Work out the finished part from the listing and answer in its coordinate system (mm). Face numbers are marked on the shaded views. A direction names the side the tool comes from. Give positions to 0.01 mm unless a question says otherwise; leave off trailing zeros. Loops run counter-clockwise (first coordinate to the right, second up) from the corner with the lowest first, then second, coordinate; pieces in that order, holes last. Notation, with made-up numbers: M 4,20.25 L 49,20.25 A24 cw 49,47.25 Z; hole C -7,43.25 d10. An arc over 180 degrees is marked long. Use a Markdown table: item, result.
```python
from build123d import *

# Parameters (mm, degrees)
CROQUIS1_W              = 70
CROQUIS1_H              = 42
SALIENTE_EXTRUIR1_DEPTH = 28
CROQUIS2_W              = 1.5
CROQUIS2_H              = 19.5
CORTAR_EXTRUIR1_DEPTH   = 70
CROQUIS3_R              = 2
CORTAR_EXTRUIR2_DEPTH   = 70
CROQUIS4_R              = 6
CORTAR_EXTRUIR3_DEPTH   = 70
CROQUIS5_R              = 10.4
CORTAR_EXTRUIR4_DEPTH   = 4.5
CROQUIS6_R              = 9.7
CROQUIS6_R_2            = 6.7
CORTAR_EXTRUIR5_DEPTH   = 1
CHAFL_N1_SIZE           = 1.2
REDONDEO1_R             = 0.7


with BuildPart() as part:
    # Croquis1 → Saliente-Extruir1 (new body)
    with BuildSketch(Plane.XY):
        Rectangle(CROQUIS1_W, CROQUIS1_H)
    extrude(amount=SALIENTE_EXTRUIR1_DEPTH)

    # Croquis2 → Cortar-Extruir1 (cut)
    with BuildSketch(Plane(origin=(35, 0, 0), x_dir=(0, 0, -1), z_dir=(1, 0, 0))):
        with Locations((-27.25, 0)):
            Rectangle(CROQUIS2_W, CROQUIS2_H)
        Polygon((0, 21), (-20, 21), (-20, 19.5), (-4.5, 19.5), (-4.5, 10.5), (0, 6), align=None)
        Polygon((-20, -19.5), (-20, -21), (0, -21), (0, -6), (-4.5, -10.5), (-4.5, -19.5), align=None)
    extrude(amount=-CORTAR_EXTRUIR1_DEPTH, mode=Mode.SUBTRACT)

    # Croquis3 → Cortar-Extruir2 (cut)
    with BuildSketch(Plane.XY.offset(28)):
        with Locations((25, -15)):
            Circle(CROQUIS3_R)
        with Locations((-25, -15)):
            Circle(CROQUIS3_R)
        with Locations((-25, 15)):
            Circle(CROQUIS3_R)
        with Locations((25, 15)):
            Circle(CROQUIS3_R)
    extrude(amount=-CORTAR_EXTRUIR2_DEPTH, mode=Mode.SUBTRACT)

    # Croquis4 → Cortar-Extruir3 (cut)
    with BuildSketch(Plane(origin=(35, 0, 0), x_dir=(0, 0, -1), z_dir=(1, 0, 0))):
        with Locations((-13, 0)):
            Circle(CROQUIS4_R)
    extrude(amount=-CORTAR_EXTRUIR3_DEPTH, mode=Mode.SUBTRACT)

    # Croquis5 → Cortar-Extruir4 (cut)
    with BuildSketch(Plane(origin=(35, 0, 0), x_dir=(0, 0, -1), z_dir=(1, 0, 0))):
        with Locations((-13, 0)):
            Circle(CROQUIS5_R)
    cortar_extruir4 = extrude(amount=-CORTAR_EXTRUIR4_DEPTH, mode=Mode.SUBTRACT)

    # Croquis6 → Cortar-Extruir5 (cut)
    with BuildSketch(Plane(origin=(30.5, 0, 0), x_dir=(0, 0, -1), z_dir=(1, 0, 0))):
        with Locations((-13, 0)):
            Circle(CROQUIS6_R)
        with Locations((-13, 0)):
            Circle(CROQUIS6_R_2, mode=Mode.SUBTRACT)
    cortar_extruir5 = extrude(amount=-CORTAR_EXTRUIR5_DEPTH, mode=Mode.SUBTRACT)

    # Simetría1: Cortar-Extruir4, Cortar-Extruir5 across plane
    add(cortar_extruir4.mirror(Plane(origin=(0, 0, 0), x_dir=(0, 0, 1), z_dir=(1, 0, 0))), mode=Mode.SUBTRACT)
    add(cortar_extruir5.mirror(Plane(origin=(0, 0, 0), x_dir=(0, 0, 1), z_dir=(1, 0, 0))), mode=Mode.SUBTRACT)

    # Chaflán1
    chafl_n1_edges = [part.edges().sort_by_distance(p)[0] for p in [
        (0, -21, 28),
        (0, -9.75, 28),
        (0, 9.75, 28),
        (0, 21, 20),
        (0, -21, 20),
        (0, 21, 28),
    ]]
    chamfer(chafl_n1_edges, length=CHAFL_N1_SIZE)

    # Redondeo1
    redondeo1_edges = [part.edges().sort_by_distance(p)[0] for p in [
        (-35, 0, 23.4),
        (35, 0, 23.4),
    ]]
    fillet(redondeo1_edges, radius=REDONDEO1_R)


solid = part.part
```
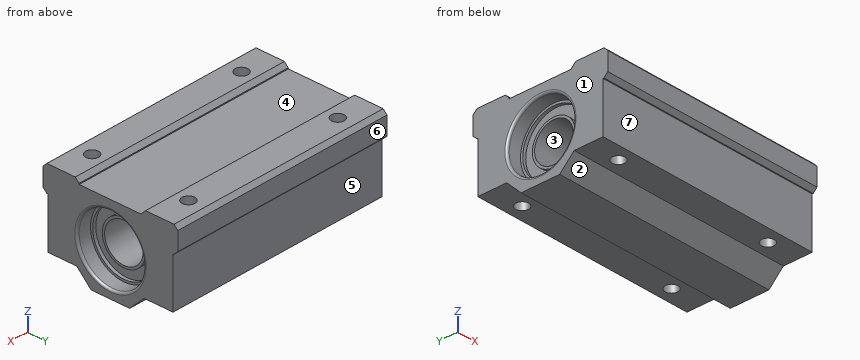
(1) Given P1, Ø4, axis at x = 12.5, y = 15, coming from the -Z side; P2, Ø16.5, axis at y = 0, z = 13, coming from the +X side; P3, Ø1.5, axis at x = 23.5, z = 18.5, coming from the +Y side, each flat-ended and moving along its own axis, determine where each tip first touches the part or whether it passes through.
Entries:
| item | result |
|---|---|
| P1 | stops at z = 4.5 |
| P2 | stops at x = 30.5 |
| P3 | stops at y = 19.5 |
(2) A cutting plane is placed at B-B (y = 15). Write down the section's boundary in (x, z).
Entries:
| item | result |
|---|---|
| outline | M -35,4.5 L -27,4.5 L -27,28 L -35,28 Z; M -23,4.5 L 23,4.5 L 23,28 L -23,28 Z; M 27,4.5 L 35,4.5 L 35,28 L 27,28 Z |
(3) A cutting plane is placed at A-A (x = -25). Count the separate pieces of the cut face and the enclosed holes in it, and give its area (3 significant figures).
Entries:
| item | result |
|---|---|
| separate pieces | 3 |
| enclosed holes | 1 |
| area | 680 mm² |
(4) A cutting plane is placed at C-C (x = 13.5). Write down the section's boundary in (y, z), and give its area (3 significant figures).
Entries:
| item | result |
|---|---|
| outline | M -21,21.2 L -19.8,20 L -19.5,20 L -19.5,4.5 L -10.5,4.5 L -6,0 L 6,0 L 10.5,4.5 L 19.5,4.5 L 19.5,20 L 19.8,20 L 21,21.2 L 21,26.8 L 19.8,28 L 10.95,28 L 9.75,26.8 L 9.75,26.5 L -9.75,26.5 L -9.75,26.8 L -10.95,28 L -19.8,28 L -21,26.8 Z; hole C 0,13 d12 |
| area | 868 mm² |
(5) Consider probe 1 along Y at (x, z) = (29.9, 13); probe 2 along X at (y, z) = (16, 20.5); probe 3 along Y at (x, z) = (25, 14.5). Determine where each line is inside the solid, lowest interval first. Write a range as [from, to].
Entries:
| item | result |
|---|---|
| probe 1 | y = [-19.5, -9.7], [-6.7, -6], [6, 6.7], [9.7, 19.5] |
| probe 2 | x = [-35, -26.73], [-23.27, 23.27], [26.73, 35] |
| probe 3 | y = [-19.5, -17], [-13, -5.81], [5.81, 13], [17, 19.5] |
(6) Which of the six approach directions +Z, -Z, +X, -X, +Y, -Y give full straight-line access (tool end or side, diameter ignored) to the marked faces 5, 6 and 7?
Entries:
| item | result |
|---|---|
| face 5 | -Z, +X, -X, +Y |
| face 6 | +Z, -Z, +X, -X, +Y |
| face 7 | -Z, +X, -X, -Y |
(7) The mould has two halves that part along Z. Classify the marked faces 1, 2, 3 and 4: released by +Z, released by -Z, zero draft, split by the parting line, or undercut.
Entries:
| item | result |
|---|---|
| face 1 | zero draft |
| face 2 | released by -Z |
| face 3 | undercut |
| face 4 | released by +Z |
